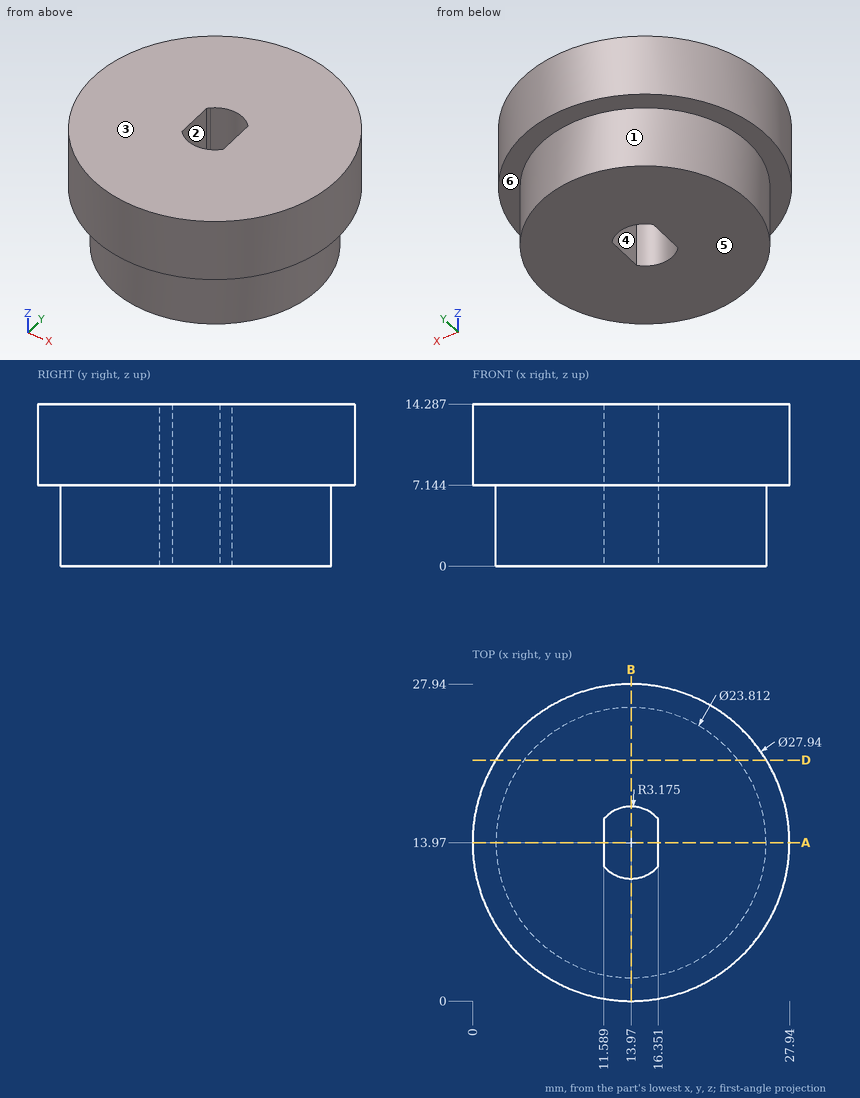
Design review of the part shown in the three views and the two pictorial views. Dimensions are in mm from the part's minimum x, y and z. A direction names the side the tool comes from. Round coordinates to 2 decimals unless told otherwise and drop trailing zeros. Write each loop counter-clockwise with the first axis right and the second up, starting at its lowest first coordinate (ties: lowest second). Pieces come first, ordered by that corner, then holes. Notation, with made-up numbers: M -3,-39 L 39,-39 A21 ccw 39,-19 Z; hole C 30.25,-11 d8. An arc over 180 degrees is marked long. Use a Markdown table: item, result. Add a question column.
Q1. To check wall thickness, follow line 1 (Z direction, x = 21, y = 24.5); line 2 (X direction, y = 7.75, z = 3); line 3 (Y direction, x = 22, z = 13.75). State the ranges of each line that lie inside material, in increasing order.
Q2. The part is to be moulded in two halves that separate along Y. For the marked faces 1, 2 and 3, say which applies: pulls with the +Y half, pulls with the -Y half, needs draft (parallel to the pull), parting line crosses it, or undercut.
Q3. We need section D-D, the plane y = 21.25. State the section outline as (x, z) points, plus the area to 3 significant figures.
Q4. We need section B-B, the plane x = 13.97. State the section outline as (y, z) points (1 decimal), plus the area to 3 significant figures.
Q5. We need section A-A, the plane y = 13.97. State the section outline as (x, z) points.
Q6. Insertion check: pin 1 (2 mm diameter, centred on x = 18, z = 6.5, fed in from -Y); pin 2 (8 mm diameter, centred on x = 19, z = 11.5, fed in from +Y); pin 3 (1.5 mm diameter, centred on x = 17, z = 10.5, fed in from +Y). Each pin has a flat end and moves straight along its axis. Give the tip position at first contact, or say it passes through.
Q7. Machinability: for the marked faces 4, 5 and 6, which of the approach directions +Z, -Z, +X, -X, +Y, -Y give a long, thin tool a straight path to every point of the face, cutting with its end or side? Answer none if there is none.
Findings below:
| question | item | result |
|---|---|---|
| 1 | line 1 | z = 7.14 to 14.29 |
| 1 | line 2 | x = 3.82 to 24.12 |
| 1 | line 3 | y = 2.54 to 25.4 |
| 2 | face 1 | parting line crosses it |
| 2 | face 2 | undercut |
| 2 | face 3 | needs draft |
| 3 | outline | M 2.05,7.14 L 4.55,7.14 L 4.55,0 L 23.39,0 L 23.39,7.14 L 25.89,7.14 L 25.89,14.29 L 2.05,14.29 Z |
| 3 | area | 305 mm² |
| 4 | outline | M 0,7.1 L 2.1,7.1 L 2.1,0 L 10.8,0 L 10.8,14.3 L 0,14.3 Z; M 17.1,0 L 25.9,0 L 25.9,7.1 L 27.9,7.1 L 27.9,14.3 L 17.1,14.3 Z |
| 4 | area | 279 mm² |
| 5 | outline | M 0,7.14 L 2.06,7.14 L 2.06,0 L 11.59,0 L 11.59,14.29 L 0,14.29 Z; M 16.35,0 L 25.88,0 L 25.88,7.14 L 27.94,7.14 L 27.94,14.29 L 16.35,14.29 Z |
| 6 | pin 1 | stops at y = 0.39 |
| 6 | pin 2 | stops at y = 27.9 |
| 6 | pin 3 | stops at y = 27.75 |
| 7 | face 4 | +Z, -Z |
| 7 | face 5 | -Z, +X, -X, +Y, -Y |
| 7 | face 6 | -Z |
